```python
from build123d import *

# Parameters (mm, degrees)
SKETCH1_R           = 1
BOSS_EXTRUDE1_DEPTH = 3.175
SKETCH2_W           = 28.35
SKETCH2_H           = 3.175
BOSS_EXTRUDE2_DEPTH = 12
SKETCH3_R           = 1.825
CUT_EXTRUDE1_DEPTH  = 3.175


with BuildPart() as part:
    # Sketch1 → Boss-Extrude1 (new body)
    with BuildSketch(Plane.XY):
        Polygon((0, 8), (0, 0), (0, -12), (28.35, -12), (28.35, 8), (23.85, 8), (23.85, 0), (4.5, 0), (4.5, 8), align=None)
        with Locations((2.75, 4)):
            Circle(SKETCH1_R, mode=Mode.SUBTRACT)
        with Locations((25.6, 4)):
            Circle(SKETCH1_R, mode=Mode.SUBTRACT)
    extrude(amount=BOSS_EXTRUDE1_DEPTH)

    # Sketch2 → Boss-Extrude2 (add)
    with BuildSketch(Plane.XY.offset(3.175)):
        with Locations((14.175, -10.4125)):
            Rectangle(SKETCH2_W, SKETCH2_H)
    extrude(amount=BOSS_EXTRUDE2_DEPTH)

    # Sketch3 → Cut-Extrude1 (cut)
    with BuildSketch(Plane(origin=(0, -8.825, 0), x_dir=(1, 0, 0), z_dir=(0, 1, 0))):
        with Locations(Location((6, -9.60325543, 0), (0, 0, 270))):
            Circle(SKETCH3_R)
        with Locations(Location((22.35, -9.60325543, 0), (0, 0, 270))):
            Circle(SKETCH3_R)
    extrude(amount=-CUT_EXTRUDE1_DEPTH, mode=Mode.SUBTRACT)


solid = part.part
```
Here's how the part is built. I have some questions about the finished solid (model axes, mm). A direction names the side the tool comes from. Give positions to 0.01 mm unless a question says otherwise; leave off trailing zeros. Write each loop counter-clockwise with the first axis right and the second up, starting at its lowest first coordinate (ties: lowest second). Pieces come first, ordered by that corner, then holes. Notation, with made-up numbers: (-10, -22) -> (22, -22) arc R8 cw to (22, -17) -> close; hole circle Ø4 at (-19.75, -34). An arc over 180 degrees is marked (long way). Write each question's results on one line, items separated by ' | '.
Item 1: For pin 1 Ø1.5 at (x, y) = (8.5, -0.5) entering from +Z (3 decimals); pin 2 Ø1 at (x, z) = (19, 2) entering from +Y; pin 3 Ø3.5 at (x, z) = (18.5, 6) entering from +Y (3 decimals), each with a flat end and sliding along its axis, tell me the tip position at first contact or that it passes through.
Output:
pin 1: stops at z = 3.175 | pin 2: stops at y = 0 | pin 3: stops at y = -8.825
Item 2: If I drill on L1, parallel to X at y = 5.5, z = 1; L2, parallel to Z at x = 7.5, y = -8 (3 decimals); L3, parallel to Y at x = 19, z = 7.5 (3 decimals), over which ranges is the centre line in solid material (lowest first)?
Output:
L1: x = 0 to 4.5, 23.85 to 28.35 | L2: z = 0 to 3.175 | L3: y = -12 to -8.825
Item 3: Suppose I cut it at C-C on x = 22.35. Write out the boundary of the cut face in (y, z) (3 decimals).
Output:
outline: (-12, 0) -> (0, 0) -> (0, 3.175) -> (-8.825, 3.175) -> (-8.825, 7.778) -> (-12, 7.778) -> close; (-12, 11.428) -> (-8.825, 11.428) -> (-8.825, 15.175) -> (-12, 15.175) -> close
Item 4: Suppose I cut it at B-B on z = 1. Write out the boundary of the cut face in (x, y).
Output:
outline: (0, -12) -> (28.35, -12) -> (28.35, 8) -> (23.85, 8) -> (23.85, 0) -> (4.5, 0) -> (4.5, 8) -> (0, 8) -> close; hole circle Ø2 at (2.75, 4); hole circle Ø2 at (25.6, 4)
Item 5: On a 3-axis mill with a long thin cutter (end or side, diameter ignored), from which of +Z, -Z, +X, -X, +Y, -Y can I reach the whole of each face in a straight line? I mean faces 1 (the face through (14, -8.825, 9)), 2 (the face through (14, 0, 2)), 3 (the face through (14, -4, 0)). Say none if no direction works.
Output:
face 1: +Z, +X, -X, +Y | face 2: +Z, -Z, +Y | face 3: -Z, +X, -X, +Y, -Y
Item 6: Suppose I cut it at A-A on y = 4. Write out the boundary of the cut face in (x, z) (3 decimals), plus the area to 3 significant figures.
Output:
outline: (0, 0) -> (1.75, 0) -> (1.75, 3.175) -> (0, 3.175) -> close; (3.75, 0) -> (4.5, 0) -> (4.5, 3.175) -> (3.75, 3.175) -> close; (23.85, 0) -> (24.6, 0) -> (24.6, 3.175) -> (23.85, 3.175) -> close; (26.6, 0) -> (28.35, 0) -> (28.35, 3.175) -> (26.6, 3.175) -> close | area: 15.9 mm^2
Item 7: We'd pull the mould along Z, two halves only. Please class faces 4 (the face through (2, 8, 2)), 5 (the face through (24.16, -10.39, 9.37)), 6 (the face through (14, -2, 3.175)): pulls with the +Z half, pulls with the -Z half, needs draft (parallel to the pull), parting line crosses it, or undercut.
Output:
face 4: needs draft | face 5: undercut | face 6: pulls with the +Z half
Item 8: Suppose I cut it at D-D on y = 1.25. Write out the boundary of the cut face in (x, z) (3 decimals), plus the area to 3 significant figures.
Output:
outline: (0, 0) -> (4.5, 0) -> (4.5, 3.175) -> (0, 3.175) -> close; (23.85, 0) -> (28.35, 0) -> (28.35, 3.175) -> (23.85, 3.175) -> close | area: 28.6 mm^2
